Part model, mm, in its own coordinate system. A direction names the side the tool comes from. Give positions to 0.01 mm unless a question says otherwise; leave off trailing zeros. Write each loop counter-clockwise with the first axis right and the second up, starting at its lowest first coordinate (ties: lowest second). Pieces come first, ordered by that corner, then holes.
from build123d import *

# Parameters (mm, degrees)
SKETCH_1_W          = 200
SKETCH_1_H          = 460
EXTRUDE_1_DEPTH     = 8
SKETCH_2_R          = 60
CUT_EXTRUDE_1_DEPTH = 10
FILLET_1_R          = 60
SKETCH_3_R          = 2.75
CUT_EXTRUDE_2_DEPTH = 10
SKETCH_4_R          = 6
CUT_EXTRUDE_3_DEPTH = 5.5
SKETCH_5_R          = 4.25
CUT_EXTRUDE_4_DEPTH = 10


with BuildPart() as part:
    # 草图1 → 凸台-拉伸1 (new body)
    with BuildSketch(Plane.XY):
        with Locations((0, 230)):
            Rectangle(SKETCH_1_W, SKETCH_1_H)
    extrude(amount=EXTRUDE_1_DEPTH)

    # 草图2 → 切除-拉伸1 (cut)
    with BuildSketch(Plane(origin=(0, 0, 0), x_dir=(-1, 0, 0), z_dir=(0, 0, -1))):
        with Locations((0, 370)):
            Circle(SKETCH_2_R)
    extrude(amount=-CUT_EXTRUDE_1_DEPTH, mode=Mode.SUBTRACT)

    # 圆角1
    fillet_1_edges = [part.edges().sort_by_distance(p)[0] for p in [
        (100, 460, 4),
        (-100, 460, 4),
    ]]
    fillet(fillet_1_edges, radius=FILLET_1_R)

    # 草图3 → 切除-拉伸2 (cut)
    with BuildSketch(Plane.XY.offset(8)):
        with Locations((27.706208015, 446.380158009)):
            Circle(SKETCH_3_R)
        with Locations((52.294053173, 432.184358988)):
            Circle(SKETCH_3_R)
        with Locations((62.184358988, 422.294053173)):
            Circle(SKETCH_3_R)
        with Locations((76.380158009, 397.706208015)):
            Circle(SKETCH_3_R)
        with Locations((76.380158009, 342.293791985)):
            Circle(SKETCH_3_R)
        with Locations((62.184358988, 317.705946827)):
            Circle(SKETCH_3_R)
        with Locations((52.294053173, 307.815641012)):
            Circle(SKETCH_3_R)
        with Locations((27.706208015, 293.619841991)):
            Circle(SKETCH_3_R)
        with Locations((-27.706208015, 293.619841991)):
            Circle(SKETCH_3_R)
        with Locations((-52.294053173, 307.815641012)):
            Circle(SKETCH_3_R)
        with Locations((-62.184358988, 317.705946827)):
            Circle(SKETCH_3_R)
        with Locations((-76.380158009, 342.293791985)):
            Circle(SKETCH_3_R)
        with Locations((-76.380158009, 397.706208015)):
            Circle(SKETCH_3_R)
        with Locations((-62.184358988, 422.294053173)):
            Circle(SKETCH_3_R)
        with Locations((-52.294053173, 432.184358988)):
            Circle(SKETCH_3_R)
        with Locations((-27.706208015, 446.380158009)):
            Circle(SKETCH_3_R)
    extrude(amount=-CUT_EXTRUDE_2_DEPTH, mode=Mode.SUBTRACT)

    # 草图4 → 切除-拉伸3 (cut)
    with BuildSketch(Plane(origin=(0, 0, 0), x_dir=(-1, 0, 0), z_dir=(0, 0, -1))):
        with Locations((27.706208015, 446.380158009)):
            Circle(SKETCH_4_R)
        with Locations((52.294053173, 432.184358988)):
            Circle(SKETCH_4_R)
        with Locations((62.184358988, 422.294053173)):
            Circle(SKETCH_4_R)
        with Locations((76.380158009, 397.706208015)):
            Circle(SKETCH_4_R)
        with Locations((76.380158009, 342.293791985)):
            Circle(SKETCH_4_R)
        with Locations((62.184358988, 317.705946827)):
            Circle(SKETCH_4_R)
        with Locations((52.294053173, 307.815641012)):
            Circle(SKETCH_4_R)
        with Locations((27.706208015, 293.619841991)):
            Circle(SKETCH_4_R)
        with Locations((-27.706208015, 293.619841991)):
            Circle(SKETCH_4_R)
        with Locations((-52.294053173, 307.815641012)):
            Circle(SKETCH_4_R)
        with Locations((-62.184358988, 317.705946827)):
            Circle(SKETCH_4_R)
        with Locations((-76.380158009, 342.293791985)):
            Circle(SKETCH_4_R)
        with Locations((-76.380158009, 397.706208015)):
            Circle(SKETCH_4_R)
        with Locations((-62.184358988, 422.294053173)):
            Circle(SKETCH_4_R)
        with Locations((-52.294053173, 432.184358988)):
            Circle(SKETCH_4_R)
        with Locations((-27.706208015, 446.380158009)):
            Circle(SKETCH_4_R)
    extrude(amount=-CUT_EXTRUDE_3_DEPTH, mode=Mode.SUBTRACT)

    # 草图5 → 切除-拉伸4 (cut)
    with BuildSketch(Plane(origin=(0, 0, 0), x_dir=(-1, 0, 0), z_dir=(0, 0, -1))):
        with Locations((40, 49)):
            Circle(SKETCH_5_R)
        with Locations((70, 49)):
            Circle(SKETCH_5_R)
        with Locations((40, 89)):
            Circle(SKETCH_5_R)
        with Locations((70, 89)):
            Circle(SKETCH_5_R)
        with Locations((40, 217)):
            Circle(SKETCH_5_R)
        with Locations((70, 177)):
            Circle(SKETCH_5_R)
        with Locations((40, 177)):
            Circle(SKETCH_5_R)
        with Locations((70, 217)):
            Circle(SKETCH_5_R)
        with Locations(Location((-70, 217, 0), (0, 0, 180))):
            Circle(SKETCH_5_R)
        with Locations(Location((-40, 177, 0), (0, 0, 180))):
            Circle(SKETCH_5_R)
        with Locations(Location((-70, 177, 0), (0, 0, 180))):
            Circle(SKETCH_5_R)
        with Locations(Location((-40, 217, 0), (0, 0, 180))):
            Circle(SKETCH_5_R)
        with Locations(Location((-70, 89, 0), (0, 0, 180))):
            Circle(SKETCH_5_R)
        with Locations(Location((-40, 89, 0), (0, 0, 180))):
            Circle(SKETCH_5_R)
        with Locations(Location((-70, 49, 0), (0, 0, 180))):
            Circle(SKETCH_5_R)
        with Locations(Location((-40, 49, 0), (0, 0, 180))):
            Circle(SKETCH_5_R)
    extrude(amount=-CUT_EXTRUDE_4_DEPTH, mode=Mode.SUBTRACT)


solid = part.part
1) Saw through at B-B (y = 370). Write the cut outline in (x, z), and give its area (3 significant figures).
Check result:
outline: (-100, 0) - (-60, 0) - (-60, 8) - (-100, 8) - close; (60, 0) - (100, 0) - (100, 8) - (60, 8) - close
area: 640 mm2
2) 3-axis set-ups, long thin cutter, end or side, ignore diameter. For faces 1 (the flat face through (-65, 316, 5.5)), 2 (the cylindrical face through (36.63, 91.59, 3.94)): which of +Z, -Z, +X, -X, +Y, -Y reach the whole face in a straight line?
Check result:
face 1: -Z
face 2: +Z, -Z
3) Saw through at D-D (z = 4). State how many separate pieces and enclosed holes the cut face has, and give its area (3 significant figures).
Check result:
separate pieces: 1
enclosed holes: 33
area: 76,400 mm2
4) Flat gauge pins, fed straight in: P1, Ø3.5, axis at x = 29, y = 444, coming from the -Z side; P2, Ø3, axis at x = -42.5, z = 3, coming from the +Y side. Where does each tip first touch, or does it go through?
Check result:
P1: stops at z = 5.5
P2: stops at y = 459.99
5) Mould opens along X. For faces 3 (the flat face through (-1, 460, 4)), 4 (the cylindrical face through (24.48, 451.44, 2.71)), 5 (the cylindrical face through (81.96, 442.89, 4.06)) say: +X half, -X half, draft (parallel to the pull), parting line (faces both ways), or undercut.
Check result:
face 3: draft
face 4: undercut
face 5: +X half
6) Saw through at C-C (x = 0). Write the cut outline in (y, z).
Check result:
outline: (0, 0) - (310, 0) - (310, 8) - (0, 8) - close; (430, 0) - (460, 0) - (460, 8) - (430, 8) - close
7) Saw through at A-A (y = 177). Write the cut outline in (x, z), and give its area (3 significant figures).
Check result:
outline: (-100, 0) - (-74.25, 0) - (-74.25, 8) - (-100, 8) - close; (-65.75, 0) - (-44.25, 0) - (-44.25, 8) - (-65.75, 8) - close; (-35.75, 0) - (35.75, 0) - (35.75, 8) - (-35.75, 8) - close; (44.25, 0) - (65.75, 0) - (65.75, 8) - (44.25, 8) - close; (74.25, 0) - (100, 0) - (100, 8) - (74.25, 8) - close
area: 1,330 mm2
8) Drill centre lines: L1, parallel to X at y = 217.5, z = 3.5; L2, parallel to Y at x = -0.5, z = 2; L3, parallel to X at y = 399.5, z = 4. Where is each one in solid material? Low to high.
Check result:
L1: x = -100 to -74.22, -65.78 to -44.22, -35.78 to 35.78, 44.22 to 65.78, 74.22 to 100
L2: y = 0 to 310, 430 to 460
L3: x = -100 to -82.11, -70.65 to -52.25, 52.25 to 70.65, 82.11 to 100
